Can you work these out from the drawing? Everything is in mm from the part's minimum corner. A direction names the side the tool comes from. Coordinates: 2 decimals unless noted, no trailing zeros. Write each loop counter-clockwise with the first axis right and the second up, starting at its lowest first coordinate (ties: lowest second). Pieces come first, ordered by that corner, then holes. Notation, with made-up numbers: (-18.75, 86.5) -> (-0.75, 86.5) arc R11 cw to (-0.75, 94.5) -> close; hole circle Ø6 at (-34, 46). An arc over 180 degrees is marked (long way). Use a Markdown table: item, result. Add a question column.
Item 1: Imagine slicing it at C-C, the plane z = 38.5. Write out the boundary of the cut face in (x, y), and give its area (3 significant figures).
Item 2: Imagine slicing it at B-B, the plane x = 36. Write out the boundary of the cut face in (y, z), and give its area (3 significant figures).
Item 3: Imagine slicing it at A-A, the plane y = 16.75. Write out the boundary of the cut face in (x, z), and give its area (3 significant figures).
Item 4: Will these pins go through, and if not, where does the flat tip stop? pin 1 Ø1.5 at (y, z) = (7, 68) entering from +X; pin 2 Ø3 at (x, y) = (13, 5) entering from +Z; pin 3 Ø8.5 at (x, y) = (14, 8) entering from -Z.
Item 5: If I drill on line 1 along Z through (x, y) = (4.5, 8.5); line 2 along Y through (x, z) = (37.5, 63), over which ranges is the centre line in solid material (lowest first)? Write a range as from..to.
Item 6: Imagine slicing it at D-D, the plane z = 6. Write out the boundary of the cut face in (x, y).
Item 7: On a 3-axis mill with a long thin cutter (end or side, diameter ignored), from which of +Z, -Z, +X, -X, +Y, -Y can I reach the whole of each face in a straight line? I mean the marked faces 1, 2, 3, 4 and 5. Say none if no direction works.
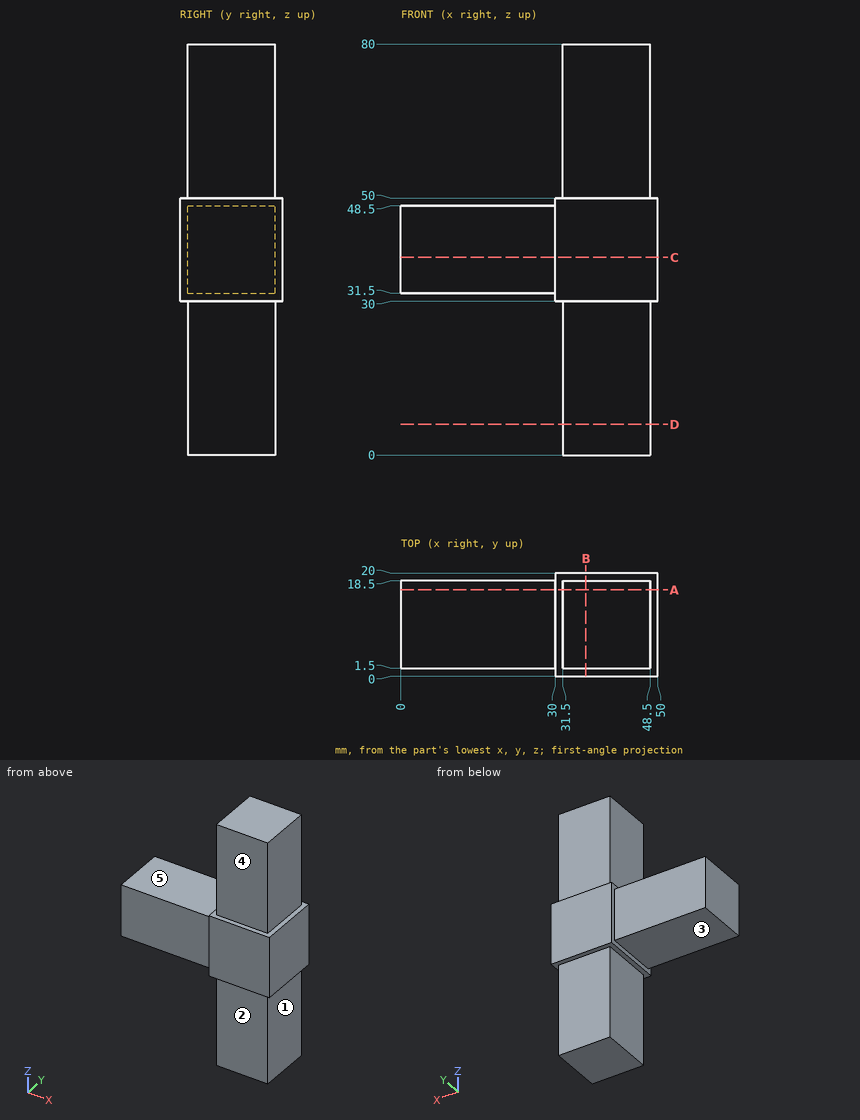
Ans:
| question | item | result |
|---|---|---|
| 1 | outline | (0, 1.5) -> (30, 1.5) -> (30, 0) -> (50, 0) -> (50, 20) -> (30, 20) -> (30, 18.5) -> (0, 18.5) -> close |
| 1 | area | 910 mm^2 |
| 2 | outline | (0, 30) -> (1.5, 30) -> (1.5, 0) -> (18.5, 0) -> (18.5, 30) -> (20, 30) -> (20, 50) -> (18.5, 50) -> (18.5, 80) -> (1.5, 80) -> (1.5, 50) -> (0, 50) -> close |
| 2 | area | 1,420 mm^2 |
| 3 | outline | (0, 31.5) -> (30, 31.5) -> (30, 30) -> (31.5, 30) -> (31.5, 0) -> (48.5, 0) -> (48.5, 30) -> (50, 30) -> (50, 50) -> (48.5, 50) -> (48.5, 80) -> (31.5, 80) -> (31.5, 50) -> (30, 50) -> (30, 48.5) -> (0, 48.5) -> close |
| 3 | area | 1,930 mm^2 |
| 4 | pin 1 | stops at x = 48.5 |
| 4 | pin 2 | stops at z = 48.5 |
| 4 | pin 3 | stops at z = 31.5 |
| 5 | line 1 | z = 31.5..48.5 |
| 5 | line 2 | y = 1.5..18.5 |
| 6 | outline | (31.5, 1.5) -> (48.5, 1.5) -> (48.5, 18.5) -> (31.5, 18.5) -> close |
| 7 | face 1 | -Z, +X, +Y, -Y |
| 7 | face 2 | -Z, +X, -X, -Y |
| 7 | face 3 | -Z, -X, +Y, -Y |
| 7 | face 4 | +Z, +X, -X, -Y |
| 7 | face 5 | +Z, -X, +Y, -Y |
